The listing builds one solid part. Answer for the finished solid, in the listing's coordinates (mm). A direction names the side the tool comes from. Round coordinates to 2 decimals unless told otherwise and drop trailing zeros. Write each loop counter-clockwise with the first axis right and the second up, starting at its lowest first coordinate (ties: lowest second). Pieces come first, ordered by that corner, then holes.
Item 1: A tool of negligible diameter and unlimited length cuts with its end or side. For faces 5 (the face through (-3, -5, 0)), 6 (the face through (0, 3.85, 4)), 7 (the face through (-10.5, 0.1, 1.6)), 8 (the face through (12.5, 0, 4)), 9 (the face through (-9, 0, 3)), from which of +Z, -Z, +X, -X, +Y, -Y can it reach the whole face along a straight path? Write none if from no direction.
Item 2: Find the intervals of material crossed by probe 1 along Y at (x, z) = (1.5, 1); probe 2 along X at (y, z) = (0.75, 2.25); probe 3 along X at (y, z) = (-2.5, 4.5), in increasing order.
Item 3: Each of these flat-tipped pins is pushed along its axis until it touches: pin 1 (0.5 mm diameter, centred on y = 0, z = 0.5, fed in from +X); pin 2 (1.2 mm diameter, centred on x = -8.5, y = 2.5, fed in from -Z). Where does it stop, or does it pass through?
Item 4: Find section B-B on x = 2.5. Give the vertices of the cut face in (y, z).
Item 5: Find section C-C on y = -0.25. Give the vertices of the cut face in (x, z).
Item 6: For a pull along X with two mould halves and no side action, classify faces 1 (the face through (0, -6, 3)), 2 (the face through (0, -3.85, 4)), 3 (the face through (-10.95, 0, 1)), 4 (the face through (-12.5, 0, 3)) as +X half, -X half, draft (parallel to the pull), parting line (faces both ways), or undercut.
Item 7: Find section D-D on z = 0.75. Give the vertices of the cut face in (x, y).
Autodesk Inventor part; units mm, degrees
ref_plane "YZ Plane" through (0, 0, 0) normal (1, 0, 0) x (0, 1, 0)
ref_plane "XZ Plane" through (0, 0, 0) normal (0, 1, 0) x (-1, 0, 0)
ref_plane "XY Plane" through (0, 0, 0) normal (0, 0, 1) x (1, 0, 0)
sketch "Sketch1" plane through (0, 0, 0) normal (0, 0, 1) x (1, 0, 0)
  line L0 (-7.15, -3.85) -> (7.15, -3.85)
  line L1 (7.15, -3.85) -> (7.15, 3.85)
  line L2 (7.15, 3.85) -> (-7.15, 3.85)
  line L3 (-7.15, 3.85) -> (-7.15, -3.85)
  line L4 (-7.15, -3.85) -> (7.15, 3.85) construction
  line L5 (7.15, -3.85) -> (-7.15, 3.85) construction
  line L6 (-12.5, -6) -> (12.5, -6)
  line L7 (12.5, -6) -> (12.5, 6)
  line L8 (12.5, 6) -> (-12.5, 6)
  line L9 (-12.5, 6) -> (-12.5, -6)
  line L10 (-12.5, -6) -> (12.5, 6) construction
  line L11 (12.5, -6) -> (-12.5, 6) construction
  point P0 (0, 0)
  dimension "d0" = 7.7
  dimension "d1" = 14.3
  dimension "d3" = 12
  dimension "d4" = 25
extrude "Extrusion1" add sketch "Sketch1" along normal blind 6.6
sketch "Sketch2" plane through (0, 0, 0) normal (0, 0, -1) x (-1, 0, 0)
  line L0 (10.15, 4.8) -> (7.15, 4.8)
  line L1 (7.15, 4.8) -> (7.15, -4.8)
  line L2 (7.15, -4.8) -> (10.15, -4.8)
  line L3 (10.15, -4.8) -> (10.15, 4.8)
  line L4 (7.15, 3.85) -> (-7.15, 3.85)
  line L5 (-7.15, -3.85) -> (7.15, -3.85)
  point P0 (0, 0)
  dimension "d8" = 3
  dimension "d18" = 9.6
  dimension "d19" = 0.95
extrude "Extrusion2" cut sketch "Sketch2" against normal blind 3
sketch "Sketch3" plane through (0, 0, 0) normal (0, 0, -1) x (-1, 0, 0)
  line L0 (17.5, 0) -> (-17.5, 0)
  line L1 (-12.65, -4.8) -> (10.95, -4.8)
  line L2 (10.95, -4.8) -> (10.95, 4.8)
  line L3 (10.95, 4.8) -> (-12.65, 4.8)
  line L4 (-12.65, 4.8) -> (-12.65, -4.8)
  line L5 (-12.65, -4.8) -> (10.95, 4.8) construction
  line L6 (10.95, -4.8) -> (-12.65, 4.8) construction
  line L7 (-7.15, 3.85) -> (-7.15, -3.85)
  line L8 (7.15, -3.85) -> (7.15, 3.85)
  line L9 (10.15, 4.8) -> (10.15, -4.8)
  point P0 (0, 0)
  point P1 (-0.85, 0)
  dimension "d13" = 5.5
  dimension "d14" = 3.8
  dimension "d15" = 9.6
extrude "Extrusion3" cut sketch "Sketch3" against normal blind 1.6
chamfer "Chamfer1" distance 0.95 angle 45 4 edges at (-7.15, 3.85, 2.3) (-7.15, -3.85, 2.3) (-10.15, -4.8, 2.3) (-10.15, 4.8, 2.3)
chamfer "Chamfer2" distance 0.5 angle 45 12 edges at (0, 3.85, 6.6) (-7.15, 0, 6.6) (0, 6, 6.6) (-12.5, 0, 6.6) (0, -6, 6.6) (12.5, 0, 6.6) (7.15, 0, 6.6) (0, -3.85, 6.6) (-12.5, 6, 3.3) (12.5, 6, 3.3) (12.5, -6, 3.3) (-12.5, -6, 3.3)
Check values:
1. face 5: -Z, +X, -X, +Y, -Y
1. face 6: +Z, -Z
1. face 7: -Z, +X
1. face 8: +Z, -Z, +X, +Y, -Y
1. face 9: -Z
2. probe 1: y = -6 to -4.8, 4.8 to 6
2. probe 2: x = -12.5 to -10.15, 7.15 to 12.5
2. probe 3: x = -12.5 to -7.15, 7.15 to 12.5
3. pin 1: stops at x = -10.95
3. pin 2: stops at z = 3
4. outline: (-6, 0) - (-4.8, 0) - (-4.8, 1.6) - (-3.85, 1.6) - (-3.85, 6.1) - (-4.35, 6.6) - (-5.5, 6.6) - (-6, 6.1) - close; (3.85, 1.6) - (4.8, 1.6) - (4.8, 0) - (6, 0) - (6, 6.1) - (5.5, 6.6) - (4.35, 6.6) - (3.85, 6.1) - close
5. outline: (-12.5, 0) - (-10.95, 0) - (-10.95, 1.6) - (-10.15, 1.6) - (-10.15, 3) - (-7.15, 3) - (-7.15, 6.1) - (-7.65, 6.6) - (-12, 6.6) - (-12.5, 6.1) - close; (7.15, 1.6) - (12.5, 1.6) - (12.5, 6.1) - (12, 6.6) - (7.65, 6.6) - (7.15, 6.1) - close
6. face 1: draft
6. face 2: undercut
6. face 3: +X half
6. face 4: -X half
7. outline: (-12.5, -5.5) - (-12, -6) - (12, -6) - (12.5, -5.5) - (12.5, -4.8) - (-10.95, -4.8) - (-10.95, 4.8) - (12.5, 4.8) - (12.5, 5.5) - (12, 6) - (-12, 6) - (-12.5, 5.5) - close
